Check sheet for the modelled part. Datum: model origin and axes. Units: mm. A direction names the side the tool comes from. Coordinates: 2 decimals unless noted, no trailing zeros. Loops run counter-clockwise (first coordinate to the right, second up) from the corner with the lowest first, then second, coordinate; pieces in that order, holes last.
from build123d import *

# Parameters (mm, degrees)
SKETCH1_R               = 5
BOSS_EXTRUDE2_DEPTH     = 7
SKETCH3_R               = 7.5
BOSS_EXTRUDE3_DEPTH     = 3
CUT_EXTRUDE1_DEPTH      = 5
CUT_EXTRUDE1_DEPTH_BACK = 5
SKETCH2_R               = 1.55
SKETCH4_R               = 3
CUT_EXTRUDE2_DEPTH      = 2.5
CUT_EXTRUDE3_START      = -2.5
SKETCH5_R               = 3
CUT_EXTRUDE3_DEPTH      = 2.5


with BuildPart() as part:
    # Sketch1 → Boss-Extrude2 (new body)
    with BuildSketch(Plane.XY):
        Circle(SKETCH1_R)
        Polygon((-3.031088913, 1.75), (0, 3.5), (3.031088913, 1.75), (3.031088913, -1.75), (0, -3.5), (-3.031088913, -1.75), align=None, mode=Mode.SUBTRACT)
    extrude(amount=BOSS_EXTRUDE2_DEPTH)

    # Sketch3 → Boss-Extrude3 (add)
    with BuildSketch(Plane.XY):
        Circle(SKETCH3_R)
    extrude(amount=BOSS_EXTRUDE3_DEPTH)

    # Sketch2 → Cut-Extrude1 (cut, two sides: drawn at the far end of the back side and taken through both)
    with BuildSketch(Plane.ZY.offset(-CUT_EXTRUDE1_DEPTH_BACK)):
        with Locations(Location((3.5, 0, 0), (0, 0, 251.180936631))):
            Circle(SKETCH2_R)
    extrude(amount=CUT_EXTRUDE1_DEPTH + CUT_EXTRUDE1_DEPTH_BACK, mode=Mode.SUBTRACT)

    # Sketch4 → Cut-Extrude2 (cut)
    with BuildSketch(Plane.ZY.offset(5)):
        with Locations((3.5, 0)):
            Circle(SKETCH4_R)
    extrude(amount=CUT_EXTRUDE2_DEPTH, mode=Mode.SUBTRACT)

    # Sketch5 → Cut-Extrude3 (cut)
    with BuildSketch(Plane.ZY.offset(-5).offset(CUT_EXTRUDE3_START)):
        with Locations((3.5, 0)):
            Circle(SKETCH5_R)
    extrude(amount=CUT_EXTRUDE3_DEPTH, mode=Mode.SUBTRACT)


solid = part.part
(1) Section check D-D, the plane x = 1. Enter the section's corners in (y, z), plus the area to 3 significant figures.
(2) Draft check along X on faces 4 (the face through (3.031, 0, 5.4)), 5 (the face through (6.93, -2.87, 1.48)), 6 (the face through (-5, 0, 1.7)), 7 (the face through (0, -2, 3)). Enter one of: pulls with the +X half, pulls with the -X half, needs draft (parallel to the pull), parting line crosses it, or undercut.
(3) Gauge pin test, flat ends, axial feed: P1, Ø2.5, axis at y = 0, z = 3.5, coming from the -X side; P2, Ø4, axis at x = 0, y = -1, coming from the +Z side; P3, Ø3, axis at y = 0, z = 4.5, coming from the -X side; P4, Ø3, axis at y = 1, z = 2, coming from the -X side. Record the tip position at first contact, or that the pin passes through.
(4) Set-up check for faces 1 (the face through (0, 2, 3)), 2 (the face through (0, -6, 3)), 3 (the face through (6.3, 0.1, 0.5)): record each of +Z, -Z, +X, -X, +Y, -Y from which the full face is reachable in a straight line by a thin tool's end or side.
(5) Section check B-B, the plane z = 6. Enter the section's corners in (x, y), plus the area to 3 significant figures.
(6) Section check A-A, the plane y = 0. Enter the section's corners in (x, z).
(7) Section check C-C, the plane x = 4.5. Enter the section's corners in (y, z), plus the area to 3 significant figures.
(8) Scan lines: line 1 along Z through (x, y) = (-1, -7); line 2 along Z through (x, y) = (0.5, 0); line 3 along X through (y, z) = (-1.75, 2.5). Record each from-to range of solid material in increasing order.
Determined:
1. outline: (-7.43, 0) - (7.43, 0) - (7.43, 3) - (4.9, 3) - (4.9, 7) - (2.92, 7) - (2.92, 3) - (1.47, 3) arc R1.55 cw to (-1.47, 3) - (-2.92, 3) - (-2.92, 7) - (-4.9, 7) - (-4.9, 3) - (-7.43, 3) - close
1. area: 58.2 mm2
2. face 4: undercut
2. face 5: parting line crosses it
2. face 6: pulls with the -X half
2. face 7: undercut
3. P1: passes through
3. P2: stops at z = 3
3. P3: stops at x = -5
3. P4: stops at x = -7.48
4. face 1: +Z
4. face 2: +Z, -Y
4. face 3: +Z, +X
5. outline: circle Ø10 at (0, 0); hole (-3.03, -1.75) - (0, -3.5) - (3.03, -1.75) - (3.03, 1.75) - (0, 3.5) - (-3.03, 1.75) - close
5. area: 46.7 mm2
6. outline: (-7.5, 0) - (7.5, 0) - (7.5, 0.5) - (5, 0.5) - (5, 1.95) - (-5, 1.95) - (-5, 0.5) - (-7.5, 0.5) - close; (-5, 5.05) - (-3.03, 5.05) - (-3.03, 7) - (-5, 7) - close; (3.03, 5.05) - (5, 5.05) - (5, 7) - (3.03, 7) - close
7. outline: (-6, 0) - (6, 0) - (6, 3) - (2.18, 3) - (2.18, 7) - (-2.18, 7) - (-2.18, 3) - (-6, 3) - close; hole circle Ø3.1 at (0, 3.5)
7. area: 45.9 mm2
8. line 1: z = 0 to 3
8. line 2: z = 0 to 1.95
8. line 3: x = -5 to 5
